```python
from build123d import *

# Parameters (mm, degrees)
SKETCH1_R           = 31.4
MAIN_CYLINDER_DEPTH = 15
INNER_SHELL_T       = -1
OUTER_BOTTOM_EDGE_R = 2
BOTTOM_HOLE_REACH   = 48.561
SKETCH10_R          = 3.5
MOUNTS_DEPTH        = 7
HOLDER_NORTH_DEPTH  = 1.6
HOLDER_SOUTH_DEPTH  = 1.6
SKETCH17_R          = 1.1
BOSS_EXTRUDE7_DEPTH = 2.5
FILLET1_R           = 0.5


with BuildPart() as part:
    # Sketch1 → Main Cylinder (new body)
    with BuildSketch(Plane(origin=(0, 0, 0), x_dir=(1, 0, 0), z_dir=(0, 1, 0))):
        with Locations(Location((0, 0, 0), (0, 0, 270))):
            Circle(SKETCH1_R)
    extrude(amount=MAIN_CYLINDER_DEPTH)

    # Inner shell
    inner_shell_openings = [part.faces().sort_by_distance(p)[0] for p in [
        (0, 15, 0),
    ]]
    offset(amount=INNER_SHELL_T, openings=inner_shell_openings, kind=Kind.INTERSECTION)

    # Outer bottom edge
    outer_bottom_edge_edges = [part.edges().sort_by_distance(p)[0] for p in [
        (0, 0, -31.4),
    ]]
    fillet(outer_bottom_edge_edges, radius=OUTER_BOTTOM_EDGE_R)

    # Sketch10 → Bottom hole (cut, up to next)
    with BuildSketch(Plane(origin=(0, 1, 0), x_dir=(-1, 0, 0), z_dir=(0, 1, 0)), mode=Mode.PRIVATE) as bottom_hole_sk1:
        with Locations(Location((0, 0, 0), (0, 0, 90))):
            Circle(SKETCH10_R)
    bottom_hole_tool1 = extrude(bottom_hole_sk1.sketch, amount=-BOTTOM_HOLE_REACH, mode=Mode.PRIVATE) & part.part
    add(bottom_hole_tool1.solids().sort_by_distance((0, 1, 0))[0], mode=Mode.SUBTRACT)

    # Sketch12 → Mounts (add)
    with BuildSketch(Plane(origin=(0, 1, 0), x_dir=(1, 0, 0), z_dir=(0, 1, 0))):
        with BuildLine():
            Line((-25.895064684, 15.925), (-12.217281253, 15.925))
            Line((-12.217281253, 15.925), (-6.409281253, 21.733))
            Line((-6.409281253, 21.733), (6.409281253, 21.733))
            Line((6.409281253, 21.733), (12.217281253, 15.925))
            Line((12.217281253, 15.925), (25.895064684, 15.925))
            ThreePointArc((25.895064684, 15.925), (0, 30.4), (-25.895064684, 15.925))
        make_face()
        with BuildLine():
            Line((-10.8458, -21.733200692), (-16.654000692, -15.925))
            Line((-16.654000692, -15.925), (-25.895064684, -15.925))
            ThreePointArc((-25.895064684, -15.925), (0, -30.4), (25.895064684, -15.925))
            Line((25.895064684, -15.925), (16.654000692, -15.925))
            Line((16.654000692, -15.925), (10.8458, -21.733200692))
            Line((10.8458, -21.733200692), (-10.8458, -21.733200692))
        make_face()
        with BuildLine():
            Line((26.8, 14.349912892), (26.8, -14.349912892))
            ThreePointArc((26.8, -14.349912892), (30.4, 0), (26.8, 14.349912892))
        make_face()
        with BuildLine():
            Line((-26.8, 14.349912892), (-26.8, -14.349912892))
            ThreePointArc((-26.8, -14.349912892), (-30.4, 0), (-26.8, 14.349912892))
        make_face()
    extrude(amount=MOUNTS_DEPTH)

    # Sketch14 → Holder (North) (add)
    with BuildSketch(Plane(origin=(0, 8, 0), x_dir=(1, 0, 0), z_dir=(0, 1, 0))):
        with BuildLine():
            Line((-20.86760348, 15.925), (-25.895064684, 15.925))
            ThreePointArc((-25.895064684, 15.925), (0, 30.4), (25.895064684, 15.925))
            Line((25.895064684, 15.925), (20.86760348, 15.925))
            ThreePointArc((20.86760348, 15.925), (0, 26.25), (-20.86760348, 15.925))
        make_face()
    extrude(amount=HOLDER_NORTH_DEPTH)

    # Sketch15 → Holder (South) (add)
    with BuildSketch(Plane(origin=(0, 8, 0), x_dir=(1, 0, 0), z_dir=(0, 1, 0))):
        with BuildLine():
            Line((-20.86760348, -15.925), (-25.895064684, -15.925))
            ThreePointArc((-25.895064684, -15.925), (0, -30.4), (25.895064684, -15.925))
            Line((25.895064684, -15.925), (20.86760348, -15.925))
            ThreePointArc((20.86760348, -15.925), (0, -26.25), (-20.86760348, -15.925))
        make_face()
    extrude(amount=HOLDER_SOUTH_DEPTH)

    # Sketch17 → Boss-Extrude7 (add)
    with BuildSketch(Plane(origin=(0, 8, 0), x_dir=(1, 0, 0), z_dir=(0, 1, 0))):
        with Locations(Location((-11.56, 20.7, 0), (0, 0, 90))):
            Circle(SKETCH17_R)
        with Locations(Location((11.56, 20.7, 0), (0, 0, 90))):
            Circle(SKETCH17_R)
    extrude(amount=BOSS_EXTRUDE7_DEPTH)

    # Fillet1
    fillet1_edges = [part.edges().sort_by_distance(p)[0] for p in [
        (11.56, 10.5, -19.6),
        (-11.56, 10.5, -19.6),
    ]]
    fillet(fillet1_edges, radius=FILLET1_R)


solid = part.part
```
Could you check a few things on this model? Use its own coordinates, in mm. A direction names the side the tool comes from. Give positions to 0.01 mm unless a question says otherwise; leave off trailing zeros. Order: outer loops, then holes, each group sorted by start corner. A loop starts at its lowest first (then second) coordinate and runs counter-clockwise, first axis right, second up.
Q1. Suppose I cut it at A-A, the plane x = 0. Write out the boundary of the cut face in (y, z).
Q2. For faces 1 (the cylindrical face through (-3.417, 0.507, -0.759)), 2 (the flat face through (0, 4, -21.733)), which set-ups out of +Z, -Z, +X, -X, +Y, -Y let a thin tool reach every point of the face, with its end or its side?
Q3. I'm going to push flat-ended pins straight in: P1, Ø5, axis at x = -8.5, z = 22.5, coming from the +Y side; P2, Ø10, axis at x = 8.5, z = 4, coming from the +Y side; P3, Ø8.5, axis at x = -9, z = -21, coming from the +Y side. Where does each tip first touch, or does it pass through?
Q4. Suppose I cut it at B-B, the plane z = 0. Write out the boundary of the cut face in (x, y), and give its area (3 significant figures).
Q5. Suppose I cut it at C-C, the plane y = 3.5. Write out the boundary of the cut face in (x, z) (3 decimals), and give its area (3 significant figures).
Q6. If I drill on line 1 along X through (y, z) = (10.75, 0); line 2 along X through (y, z) = (6.5, -11); line 3 along Y through (x, z) = (-17.5, 20), over which ranges is the centre line in solid material (lowest first)?
Solution:
1. outline: (0, -29.4) arc R2 ccw to (2, -31.4) - (15, -31.4) - (15, -30.4) - (9.6, -30.4) - (9.6, -26.25) - (8, -26.25) - (8, -21.73) - (1, -21.73) - (1, -3.5) - (0, -3.5) - close; (0, 3.5) - (1, 3.5) - (1, 21.73) - (8, 21.73) - (8, 26.25) - (9.6, 26.25) - (9.6, 30.4) - (15, 30.4) - (15, 31.4) - (2, 31.4) arc R2 ccw to (0, 29.4) - close
2. face 1: +Y, -Y
2. face 2: +Y
3. P1: stops at y = 9.6
3. P2: stops at y = 1
3. P3: stops at y = 10.5
4. outline: (-31.4, 2) arc R2 ccw to (-29.4, 0) - (-3.5, 0) - (-3.5, 1) - (-26.8, 1) - (-26.8, 8) - (-30.4, 8) - (-30.4, 15) - (-31.4, 15) - close; (3.5, 0) - (29.4, 0) arc R2 ccw to (31.4, 2) - (31.4, 15) - (30.4, 15) - (30.4, 8) - (26.8, 8) - (26.8, 1) - (3.5, 1) - close
4. area: 132 mm2
5. outline: circle Ø62.8 at (0, 0); hole (-26.8, -14.35) arc R30.4 ccw to (-25.895, -15.925) - (-12.217, -15.925) - (-6.409, -21.733) - (6.409, -21.733) - (12.217, -15.925) - (25.895, -15.925) arc R30.4 ccw to (26.8, -14.35) - (26.8, 14.35) arc R30.4 ccw to (25.895, 15.925) - (16.654, 15.925) - (10.846, 21.733) - (-10.846, 21.733) - (-16.654, 15.925) - (-25.895, 15.925) arc R30.4 ccw to (-26.8, 14.35) - close
5. area: 1,130 mm2
6. line 1: x = -31.4 to -30.4, 30.4 to 31.4
6. line 2: x = -29.41 to -26.8, 26.8 to 29.41
6. line 3: y = 0 to 9.6
